Verification items for the finished model (mm, model axes). A direction names the side the tool comes from. Coordinates: 2 decimals unless noted, no trailing zeros. Order: outer loops, then holes, each group sorted by start corner. A loop starts at its lowest first (then second) coordinate and runs counter-clockwise, first axis right, second up. Notation, with made-up numbers: M 23.25,25 L 82.25,25 A11 cw 82.25,37 Z; hole C 47,56 d9. An arc over 180 degrees is marked long. Return JSON: item names as keys, results as strings. Group by question number.
Q1. Thickness scan on probe 1 along Y at (x, z) = (8.5, -15.5); probe 2 along X at (y, z) = (54.5, -19); probe 3 along Y at (x, z) = (-17, -28.25). Record the ranges inside material, lowest first.
Q2. Section check B-B, the plane y = 40. Enter the section's corners in (x, z).
Q3. Section check C-C, the plane x = 3.5. Enter the section's corners in (y, z), then the cut area to 3 significant figures.
Q4. Mould release check, pull along Z, two halves, no side actions. Record for faces 5 (the face through (-44.6, 58.7, -12.839)), 6 (the face through (-7.071, 11, -11)), 7 (the face through (11.249, 28, -20)): pulls with the +Z half, pulls with the -Z half, needs draft (parallel to the pull), parting line crosses it, or undercut.
Q5. Section check A-A, the plane z = -29. Enter the section's corners in (x, y), then the cut area to 3 significant figures.
Q6. Access from +Z, -Z, +X, -X, +Y, -Y to the whole of each face (thin tool, end or side, straight path). Record for faces 1 (the face through (-40.807, 28, -20)), 2 (the face through (-9.817, 0.575, -20.324)), 3 (the face through (-16, 1, -14.063)), 4 (the face through (-12.06, 24.64, -14.79)).
Q7. Go/stop test with flat-tipped pins: pin 1 Ø12 at (y, z) = (32, -24) entering from +X; pin 2 Ø5 at (x, z) = (-23, -22.5) entering from -Y; pin 3 Ø12 at (x, z) = (-11.5, -29) entering from +Y; pin 4 Ø2.5 at (x, y) = (-13, 6.5) entering from -Z. Record where each tip stops, or that it passes through.
Q8. Section check D-D, the plane x = 16.5. Enter the section's corners in (y, z), then the cut area to 3 significant figures.
from build123d import *

# Parameters (mm, degrees)
SKETCH6_W            = 10.1981
SKETCH6_H            = 6.43128
BOSS_EXTRUDE3_DEPTH  = 25.4
SKETCH8_R            = 5.09905
BOSS_EXTRUDE5_DEPTH  = 12.7
SKETCH11_W           = 65.69456
SKETCH11_H           = 25.654
SKETCH11_W_2         = 6.368021248
SKETCH11_H_2         = 20.557169264
SKETCH11_W_3         = 6.453498043
SKETCH11_H_3         = 19.787878106
BOSS_EXTRUDE10_DEPTH = 4.28752
SKETCH16_W           = 1.143
SKETCH16_H           = 10.16
BOSS_EXTRUDE11_DEPTH = 38.0746
SKETCH17_W           = 26.52268
SKETCH17_H           = 10.16
BOSS_EXTRUDE12_DEPTH = 2.2606
FILLET2_R            = 2.54
FILLET3_R            = 2.54
FILLET4_R            = 2.54
SKETCH19_R           = 4.064
CUT_EXTRUDE1_DEPTH   = 12.7


with BuildPart() as part:
    # Sketch6 → Boss-Extrude3 (new body)
    with BuildSketch(Plane(origin=(0, 0, 0), x_dir=(1, 0, 0), z_dir=(0, 1, 0))):
        with Locations((-12.169797761, 10.84768804)):
            Rectangle(SKETCH6_W, SKETCH6_H)
    extrude(amount=BOSS_EXTRUDE3_DEPTH)

    # Sketch8 → Boss-Extrude5 (add)
    with BuildSketch(Plane.XY.offset(-14.06332804)):
        with Locations((-12.169797761, 5.098542)):
            Circle(SKETCH8_R)
    extrude(amount=-BOSS_EXTRUDE5_DEPTH)

    # Sketch11 → Boss-Extrude10 (add)
    with BuildSketch(Plane(origin=(0, 25.4, 0), x_dir=(1, 0, 0), z_dir=(0, 1, 0))):
        with Locations((-12.150747761, 20.45904804)):
            Rectangle(SKETCH11_W, SKETCH11_H)
        with Locations((-37.622832753, 20.159879257)):
            Rectangle(SKETCH11_W_2, SKETCH11_H_2, mode=Mode.SUBTRACT)
        with Locations((14.475273968, 20.031664064)):
            Rectangle(SKETCH11_W_3, SKETCH11_H_3, mode=Mode.SUBTRACT)
    extrude(amount=BOSS_EXTRUDE10_DEPTH)

    # Sketch16 → Boss-Extrude11 (add)
    with BuildSketch(Plane(origin=(0, 29.68752, 0), x_dir=(1, 0, 0), z_dir=(0, 1, 0))):
        with Locations((-44.426527761, 17.91904804)):
            Rectangle(SKETCH16_W, SKETCH16_H)
        with Locations((20.125032239, 17.91904804)):
            Rectangle(SKETCH16_W, SKETCH16_H)
    extrude(amount=BOSS_EXTRUDE11_DEPTH)

    # Sketch17 → Boss-Extrude12 (add)
    with BuildSketch(Plane(origin=(0, 67.76212, 0), x_dir=(1, 0, 0), z_dir=(0, 1, 0))):
        with Locations((-31.736687761, 17.91904804)):
            Rectangle(SKETCH17_W, SKETCH17_H)
        with Locations((7.435192239, 17.91904804)):
            Rectangle(SKETCH17_W, SKETCH17_H)
    extrude(amount=BOSS_EXTRUDE12_DEPTH)

    # Fillet2
    fillet2_edges = [part.edges().sort_by_distance(p)[0] for p in [
        (-12.169797761, 25.4, -14.06332804),
    ]]
    fillet(fillet2_edges, radius=FILLET2_R)

    # Fillet3
    fillet3_edges = [part.edges().sort_by_distance(p)[0] for p in [
        (-17.268847761, 25.4, -12.11768804),
    ]]
    fillet(fillet3_edges, radius=FILLET3_R)

    # Fillet4
    fillet4_edges = [part.edges().sort_by_distance(p)[0] for p in [
        (-7.070747761, 25.4, -12.11768804),
    ]]
    fillet(fillet4_edges, radius=FILLET4_R)

    # Sketch19 → Cut-Extrude1 (cut)
    with BuildSketch(Plane(origin=(0, 0, -26.76332804), x_dir=(-1, 0, 0), z_dir=(0, 0, -1))):
        with Locations((12.169797761, 5.098542)):
            Circle(SKETCH19_R)
    extrude(amount=-CUT_EXTRUDE1_DEPTH, mode=Mode.SUBTRACT)


solid = part.part
Numbers:
{
 "1": {"probe 1": "y = 25.4 to 29.69, 67.76 to 70.02", "probe 2": "x = -45 to -43.86, 19.55 to 20.7", "probe 3": "y = 25.4 to 29.69"},
 "2": {"outline": "M -45,-23 L -43.86,-23 L -43.86,-12.84 L -45,-12.84 Z; M 19.55,-23 L 20.7,-23 L 20.7,-12.84 L 19.55,-12.84 Z"},
 "3": {"outline": "M 25.4,-33.29 L 29.69,-33.29 L 29.69,-7.63 L 25.4,-7.63 Z; M 67.76,-23 L 70.02,-23 L 70.02,-12.84 L 67.76,-12.84 Z", "area": "133 mm2"},
 "4": {"face 5": "pulls with the +Z half", "face 6": "needs draft", "face 7": "undercut"},
 "5": {"outline": "M -45,25.4 L -40.81,25.4 L -40.81,29.69 L -45,29.69 Z; M -34.44,25.4 L 11.25,25.4 L 11.25,29.69 L -34.44,29.69 Z; M 17.7,25.4 L 20.7,25.4 L 20.7,29.69 L 17.7,29.69 Z", "area": "227 mm2"},
 "6": {"face 1": "-Y", "face 2": "-Z", "face 3": "-Z, -X, -Y", "face 4": "-Z, +X, -X"},
 "7": {"pin 1": "stops at x = 20.7", "pin 2": "stops at y = 25.4", "pin 3": "stops at y = 29.69", "pin 4": "stops at z = -14.06"},
 "8": {"outline": "M 25.4,-33.29 L 29.69,-33.29 L 29.69,-29.93 L 25.4,-29.93 Z; M 25.4,-10.14 L 29.69,-10.14 L 29.69,-7.63 L 25.4,-7.63 Z; M 67.76,-23 L 70.02,-23 L 70.02,-12.84 L 67.76,-12.84 Z", "area": "48.1 mm2"}
}
